```python
from build123d import *

# Parameters (mm, degrees)
F0_R     = 22.5
F1_DEPTH = 4
F2_R     = 2
F4_R     = 0.2
F5_R     = 12.5
F6_DEPTH = 4


# Not quite as in the source:
# - a fillet or chamfer that OpenCascade refuses, or shapes differently, is made with other operations: its cross-section is extruded or revolved along the edge and cut away or added


with BuildPart() as f1:
    # F0 (on Top) → F1 (new body)
    with BuildSketch(Plane.XY):
        Circle(F0_R)
        with BuildLine():
            ThreePointArc((2.2360679775, 2), (2.8025170769, 1.0704662693), (3, 0))
            ThreePointArc((3, 0), (2.8025170769, -1.0704662693), (2.2360679775, -2))
            ThreePointArc((2.2360679775, -2), (0, -3), (-2.2360679775, -2))
            ThreePointArc((-2.2360679775, -2), (-3, 0), (-2.2360679775, 2))
            ThreePointArc((-2.2360679775, 2), (0, 3), (2.2360679775, 2))
        make_face(mode=Mode.SUBTRACT)
        with BuildLine():
            ThreePointArc((-2.2360679775, -2), (0, -3), (2.2360679775, -2))
            Line((2.2360679775, -2), (-2.2360679775, -2))
        make_face()
        with BuildLine():
            Line((-2.2360679775, 2), (2.2360679775, 2))
            ThreePointArc((2.2360679775, 2), (0, 3), (-2.2360679775, 2))
        make_face()
    extrude(amount=F1_DEPTH)

    # F2 (on Front) → F3 (revolve, cut)
    with BuildSketch(Plane.XZ):
        with Locations((-23.5, 2)):
            Circle(F2_R)
    revolve(axis=Axis((0, 0, 4), (0, 0, 1)), mode=Mode.SUBTRACT)

    # F4
    f4_edges = [f1.edges().sort_by_distance(p)[0] for p in [
        (-22.5, 0, 4),
        (-22.5, 0, 0),
    ]]
    fillet(f4_edges, radius=F4_R)

    # F5 (on face) → F6 (join)
    with BuildSketch(Plane.XY.offset(4)):
        Circle(F5_R)
        with BuildLine():
            Line((2.2360679775, -2), (-2.2360679775, -2))
            ThreePointArc((-2.2360679775, -2), (-3, 0), (-2.2360679775, 2))
            Line((-2.2360679775, 2), (2.2360679775, 2))
            ThreePointArc((2.2360679775, 2), (3, 0), (2.2360679775, -2))
        make_face(mode=Mode.SUBTRACT)
    extrude(amount=F6_DEPTH)

    # F7: chamfer of 5 on 1 edges, made by hand


with BuildPart() as f7_tool2:
    # F7_s3 → F7_t4 (revolve)
    with BuildSketch(Plane.XZ):
        Polygon((7.5, 8), (12.5, 3), (12.5, 8), align=None)
    revolve(axis=Axis((0, 0, 8), (0, 0, 1)))

    split(bisect_by=Plane.XY.offset(4), keep=Keep.TOP)


with BuildPart() as f1_1:
    add(f1.part)

    # F7_t1: cut F7_tool2
    add(f7_tool2.part, mode=Mode.SUBTRACT)


solid = f1_1.part
```
Part model, mm, in its own coordinate system. A direction names the side the tool comes from. Give positions to 0.01 mm unless a question says otherwise; leave off trailing zeros. Order: outer loops, then holes, each group sorted by start corner. A loop starts at its lowest first (then second) coordinate and runs counter-clockwise, first axis right, second up. Notation, with made-up numbers: M 5.5,-31 L 22.5,-31 A25 ccw 22.5,6 Z; hole C 0,49.5 d6. An arc over 180 degrees is marked long. Use a Markdown table: item, result. Add a question column.
(1) Drop flat-ended pins along their axis: P1, Ø2, axis at y = 17, z = 3, coming from the +X side; P2, Ø4, axis at x = 10.5, y = 8, coming from the +Z side; P3, Ø1.5, axis at x = -11.5, y = -1.5, coming from the +Z side; P4, Ø1.5, axis at y = 14, z = 5.5, coming from the -X side. Give the stop position or say it passes through.
(2) 3-axis set-ups, long thin cutter, end or side, ignore diameter. For faces 1 (the face through (10, -10, 4)), 2 (the face through (0, -5, 0)), 3 (the face through (0, -2, 4)): which of +Z, -Z, +X, -X, +Y, -Y reach the whole face in a straight line?
(3) Saw through at A-A, the plane x = 0. Give the cut face in (y, z).
(4) Saw through at B-B, the plane z = 5. Give the cut face in (x, y).
(5) Mould opens along Y. For faces 4 (the face through (3.2, 0.1, 8)), 5 (the face through (7.39, 2.33, 7.75)), 6 (the face through (0, 2, 4)) say: +Y half, -Y half, draft (parallel to the pull), parting line (faces both ways), or undercut.
(6) Probe line 1 along Z through (x, y) = (-15.5, 5); line 2 along X through (y, z) = (1, 5.75); line 3 along Y through (x, z) = (-2.5, 4.75). List the from-to ranges inside material, lowest first. Write a range as [from, to].
Answer key:
| question | item | result |
|---|---|---|
| 1 | P1 | x = 15.49 |
| 1 | P2 | z = 4.3 |
| 1 | P3 | z = 4.65 |
| 1 | P4 | through |
| 2 | face 1 | +Z |
| 2 | face 2 | -Z, +X, -X, +Y, -Y |
| 2 | face 3 | +Z, -Z |
| 3 | outline | M -22.5,0.2 A0.2 ccw -22.3,0 L -2,0 L -2,8 L -7.5,8 L -11.5,4 L -22.3,4 A0.2 ccw -22.5,3.8 L -22.5,3.73 A2 cw -22.5,0.27 Z; M 2,0 L 22.3,0 A0.2 ccw 22.5,0.2 L 22.5,0.27 A2 cw 22.5,3.73 L 22.5,3.8 A0.2 ccw 22.3,4 L 11.5,4 L 7.5,8 L 2,8 Z |
| 4 | outline | C 0,0 d21; hole M -2.24,-2 L 2.24,-2 A3 ccw 2.24,2 L -2.24,2 A3 ccw Z |
| 5 | face 4 | draft |
| 5 | face 5 | parting line |
| 5 | face 6 | undercut |
| 6 | line 1 | [0, 4] |
| 6 | line 2 | [-9.7, -2.83], [2.83, 9.7] |
| 6 | line 3 | [-10.46, -1.66], [1.66, 10.46] |
